```python
from build123d import *

# Parameters (mm, degrees)
F0_R     = 4.445
F1_DEPTH = 4.7625


# Not quite as in the source:
# - a length typed as a fraction of an inch, garbled in the dataset ("3 / 203.2 mm" for 3/8 in), is restored


with BuildPart() as f1:
    # F0 (on Top) → F1 (new body)
    with BuildSketch(Plane.XY):
        Circle(F0_R)
        with BuildLine():
            ThreePointArc((2.286, 2.5044773527), (3.1024023119, 1.3686864889), (3.3909, 0))
            ThreePointArc((3.3909, 0), (3.1024023119, -1.3686864889), (2.286, -2.5044773527))
            ThreePointArc((2.286, -2.5044773527), (0, -3.3909), (-2.286, -2.5044773527))
            ThreePointArc((-2.286, -2.5044773527), (-3.3909, 0), (-2.286, 2.5044773527))
            ThreePointArc((-2.286, 2.5044773527), (0, 3.3909), (2.286, 2.5044773527))
        make_face(mode=Mode.SUBTRACT)
        with BuildLine():
            Line((-2.286, -2.5044773527), (-2.286, 2.5044773527))
            ThreePointArc((-2.286, 2.5044773527), (-3.3909, 0), (-2.286, -2.5044773527))
        make_face()
        with BuildLine():
            ThreePointArc((2.286, -2.5044773527), (3.1024023119, -1.3686864889), (3.3909, 0))
            ThreePointArc((3.3909, 0), (3.1024023119, 1.3686864889), (2.286, 2.5044773527))
            Line((2.286, 2.5044773527), (2.286, -2.5044773527))
        make_face()
    extrude(amount=F1_DEPTH)


solid = f1.part
```
Source: CAD feature listing. Evaluate the final solid. Frame: model axes, mm. A direction names the side the tool comes from. Round coordinates to 2 decimals unless told otherwise and drop trailing zeros. Loops run counter-clockwise (first coordinate to the right, second up) from the corner with the lowest first, then second, coordinate; pieces in that order, holes last.
1. Contact query for a flat-ended pin moving along its axis: pin 1 (1.5 mm diameter, centred on x = 3.5, z = 3.5, fed in from -Y). Output: stop coordinate, or through.
2. Section query B-B on y = 0. Output: boundary loops of the cut face in (x, z) (1 decimal), and give its area (3 significant figures).
3. Access query for faces 5 (the flat face through (-2.286, 0, 2)), 6 (the flat face through (3, 0, 0)). Directions: +Z, -Z, +X, -X, +Y, -Y. A direction counts if a zero-diameter tool reaches every point of the face in a straight line with its end or side. Return the directions, or none.
4. Mould query, pull axis X, two halves, no side actions, for faces 1 (the cylindrical face through (0.04, -3.39, 2.35)), 2 (the flat face through (2.286, 0, 2)), 3 (the flat face through (3, 0, 4.762)), 4 (the cylindrical face through (-0.96, -4.34, 2.35)). Classes: released by +X, released by -X, zero draft, split by the parting line, or undercut.
5. Ray query, L1, parallel to Y at x = 0.25, z = 4.45; L2, parallel to X at y = -0.5, z = 3.3; L3, parallel to X at y = -3, z = 2.1. Return the intervals inside material, ascending.
6. Section query A-A on x = 0. Output: boundary loops of the cut face in (y, z) (1 decimal), and give its area (3 significant figures).
7. Section query C-C on z = 2.9. Output: boundary loops of the cut face in (x, y) (3 decimals), and give its area (3 significant figures).
8. Section query D-D on x = -2.75. Output: boundary loops of the cut face in (y, z), and give its area (3 significant figures).
Answers below:
1. pin 1: stops at y = -3.49
2. outline: (-4.4, 0) - (-2.3, 0) - (-2.3, 4.8) - (-4.4, 4.8) - close; (2.3, 0) - (4.4, 0) - (4.4, 4.8) - (2.3, 4.8) - close
2. area: 20.6 mm2
3. face 5: +Z, -Z
3. face 6: -Z, +X, -X, +Y, -Y
4. face 1: undercut
4. face 2: undercut
4. face 3: zero draft
4. face 4: split by the parting line
5. L1: y = -4.44 to -3.38, 3.38 to 4.44
5. L2: x = -4.42 to -2.29, 2.29 to 4.42
5. L3: x = -3.28 to -1.58, 1.58 to 3.28
6. outline: (-4.4, 0) - (-3.4, 0) - (-3.4, 4.8) - (-4.4, 4.8) - close; (3.4, 0) - (4.4, 0) - (4.4, 4.8) - (3.4, 4.8) - close
6. area: 10.0 mm2
7. outline: circle Ø8.89 at (0, 0); hole (-2.286, -2.504) arc R3.391 ccw to (2.286, -2.504) - (2.286, 2.504) arc R3.391 ccw to (-2.286, 2.504) - close
7. area: 33.6 mm2
8. outline: (-3.49, 0) - (3.49, 0) - (3.49, 4.76) - (-3.49, 4.76) - close
8. area: 33.3 mm2
